from build123d import *

# Parameters (mm, degrees)
BOSS_EXTRUDE1_DEPTH = 5
SKETCH2_W           = 3.3
SKETCH2_H           = 6
CUT_EXTRUDE2_DEPTH  = 6.5
SKETCH3_R           = 2.15
CUT_EXTRUDE4_DEPTH  = 24
FILLET1_R           = 0.5
FILLET2_R           = 3
SKETCH5_W           = 10.2
SKETCH5_H           = 7
CUT_EXTRUDE5_DEPTH  = 44.231932642
SKETCH8_W           = 20
SKETCH8_H           = 7
CUT_EXTRUDE6_DEPTH  = 44.231932642
SKETCH9_W           = 20
SKETCH9_H           = 7
BOSS_EXTRUDE2_DEPTH = 10
SKETCH10_R          = 2.55
CUT_EXTRUDE7_DEPTH  = 45.955533586
FILLET3_R           = 5
SKETCH11_W          = 40
SKETCH11_H          = 10
BOSS_EXTRUDE3_DEPTH = 10
SKETCH13_W          = 35.742737896
SKETCH13_H          = 10
BOSS_EXTRUDE5_DEPTH = 5
SKETCH14_R          = 1.4
CUT_EXTRUDE8_DEPTH  = 47.75467891
SKETCH16_W          = 20
SKETCH16_H          = 3
CUT_EXTRUDE10_DEPTH = 5
SKETCH17_R          = 1
CUT_EXTRUDE11_DEPTH = 3.5


with BuildPart() as part:
    # Sketch1 → Boss-Extrude1 (new, symmetric)
    with BuildSketch(Plane.XY):
        with BuildLine():
            Line((40, -13), (34.35, -13))
            Line((34.35, -13), (34.35, 3))
            ThreePointArc((34.35, 3), (26.182605601, 5.085665361), (32.35, -0.660601044))
            Line((32.35, -0.660601044), (32.35, -13))
            Line((32.35, -13), (7.5, -13))
            Line((7.5, -13), (7.5, -6))
            Line((7.5, -6), (5.1, -6))
            Line((5.1, -6), (5.1, -13))
            Line((5.1, -13), (-5.1, -13))
            Line((-5.1, -13), (-5.1, -6))
            Line((-5.1, -6), (-7.5, -6))
            Line((-7.5, -6), (-7.5, -13))
            Line((-7.5, -13), (-32.35, -13))
            Line((-32.35, -13), (-32.35, -0.660601044))
            ThreePointArc((-32.35, -0.660601044), (-26.182605601, 5.085665361), (-34.35, 3))
            Line((-34.35, 3), (-34.35, -13))
            Line((-34.35, -13), (-40, -13))
            Line((-40, -13), (-40, 13))
            Line((-40, 13), (40, 13))
            Line((40, 13), (40, -13))
        make_face()
    extrude(amount=BOSS_EXTRUDE1_DEPTH, both=True)

    # Sketch2 → Cut-Extrude2 (cut)
    with BuildSketch(Plane.XY.offset(5)):
        with Locations((-24, -10)):
            Rectangle(SKETCH2_W, SKETCH2_H)
        with Locations((24, -10)):
            Rectangle(SKETCH2_W, SKETCH2_H)
    extrude(amount=-CUT_EXTRUDE2_DEPTH, mode=Mode.SUBTRACT)

    # Sketch3 → Cut-Extrude4 (cut)
    with BuildSketch(Plane.ZY.offset(40)):
        with Locations(Location((2, -10, 0), (0, 0, 90))):
            Circle(SKETCH3_R)
    cut_extrude4 = extrude(amount=-CUT_EXTRUDE4_DEPTH, mode=Mode.SUBTRACT)

    # Mirror1: Cut-Extrude4 across plane
    add(cut_extrude4.mirror(Plane(origin=(0, 0, 0), x_dir=(0, 0, 1), z_dir=(1, 0, 0))), mode=Mode.SUBTRACT)

    # Fillet1
    fillet1_edges = [part.edges().sort_by_distance(p)[0] for p in [
        (5.1, -9.5, -5),
        (-5.1, -9.5, -5),
    ]]
    fillet(fillet1_edges, radius=FILLET1_R)

    # Fillet2
    fillet2_edges = [part.edges().sort_by_distance(p)[0] for p in [
        (-40, 13, 0),
        (40, 13, 0),
    ]]
    fillet(fillet2_edges, radius=FILLET2_R)

    # Sketch5 → Cut-Extrude5 (cut, through all)
    with BuildSketch(Plane.XY.offset(5)):
        with Locations((0, -9.5)):
            Rectangle(SKETCH5_W, SKETCH5_H)
    extrude(amount=-CUT_EXTRUDE5_DEPTH, mode=Mode.SUBTRACT)

    # Sketch8 → Cut-Extrude6 (cut, through all)
    with BuildSketch(Plane(origin=(0, 0, -5), x_dir=(-1, 0, 0), z_dir=(0, 0, -1))):
        with Locations((0, -9.5)):
            Rectangle(SKETCH8_W, SKETCH8_H)
    extrude(amount=-CUT_EXTRUDE6_DEPTH, mode=Mode.SUBTRACT)

    # Sketch9 → Boss-Extrude2 (add)
    with BuildSketch(Plane.XY.offset(5)):
        with Locations((0, -2.5)):
            Rectangle(SKETCH9_W, SKETCH9_H)
    extrude(amount=BOSS_EXTRUDE2_DEPTH)

    # Sketch10 → Cut-Extrude7 (cut, through all)
    with BuildSketch(Plane(origin=(0, 1, 0), x_dir=(1, 0, 0), z_dir=(0, 1, 0))):
        with Locations(Location((0, -9.5, 0), (0, 0, 270))):
            Circle(SKETCH10_R)
    extrude(amount=-CUT_EXTRUDE7_DEPTH, mode=Mode.SUBTRACT)

    # Fillet3
    fillet3_edges = [part.edges().sort_by_distance(p)[0] for p in [
        (-10, -2.5, 15),
        (10, -2.5, 15),
    ]]
    fillet(fillet3_edges, radius=FILLET3_R)

    # Sketch11 → Boss-Extrude3 (add)
    with BuildSketch(Plane(origin=(0, 0, -5), x_dir=(-1, 0, 0), z_dir=(0, 0, -1))):
        with Locations((0, -1)):
            Rectangle(SKETCH11_W, SKETCH11_H)
    extrude(amount=BOSS_EXTRUDE3_DEPTH)

    # Sketch13 → Boss-Extrude5 (add)
    with BuildSketch(Plane.XZ.offset(13)):
        Rectangle(SKETCH13_W, SKETCH13_H)
    extrude(amount=BOSS_EXTRUDE5_DEPTH)

    # Sketch14 → Cut-Extrude8 (cut, through all)
    with BuildSketch(Plane.XZ.offset(6)):
        with Locations((-15, -10)):
            Circle(SKETCH14_R)
        with Locations(Location((15, -10, 0), (0, 0, 270))):
            Circle(SKETCH14_R)
    extrude(amount=-CUT_EXTRUDE8_DEPTH, mode=Mode.SUBTRACT)

    # Sketch16 → Cut-Extrude10 (cut)
    with BuildSketch(Plane.XY.offset(5)):
        with Locations((0, -14.5)):
            Rectangle(SKETCH16_W, SKETCH16_H)
    extrude(amount=-CUT_EXTRUDE10_DEPTH, mode=Mode.SUBTRACT)

    # Sketch17 → Cut-Extrude11 (cut)
    with BuildSketch(Plane.XZ.offset(18)):
        with Locations((-13.871368948, 0)):
            Circle(SKETCH17_R)
        with Locations(Location((13.871368948, 0, 0), (0, 0, 180))):
            Circle(SKETCH17_R)
    extrude(amount=-CUT_EXTRUDE11_DEPTH, mode=Mode.SUBTRACT)


solid = part.part
Design review of the part built by this model. Coordinates are the model's own, in mm. A direction names the side the tool comes from. Round coordinates to 2 decimals unless told otherwise and drop trailing zeros. Loops run counter-clockwise (first coordinate to the right, second up) from the corner with the lowest first, then second, coordinate; pieces in that order, holes last. Notation, with made-up numbers: (-29, 28.25) - (-4, 28.25) arc R29 cw to (-4, 62.25) - close; hole circle Ø4 at (-39, 0). An arc over 180 degrees is marked (long way). One line per item, written item: value. Start each with the question number.
1) Draft analysis for pull direction X (two halves, no side actions). For faces 1 (the cylindrical face through (-15.303, -1.07, -11.367)), 2 (the cylindrical face through (39.14, 12.1, 0.07)), 3 (the flat face through (-40, -2, 0)), state which applies: +X half, -X half, draft (parallel to the pull), parting line (faces both ways), or undercut.
2) To check wall thickness, follow L1, parallel to Z at x = 30, y = -10; L2, parallel to X at y = -3.5, z = 1.75; L3, parallel to Y at x = -8, z = -1.75. State the ranges of each line that lie inside material, in increasing order. Write a range as from..to.
3) Consider section A-A on x = 30. Give the boundary of the cut face in (y, z), then the cut area to 3 significant figures.
4) Insertion check: pin 1 Ø1 at (x, z) = (1.5, 11.5) entering from +Y; pin 2 Ø3.5 at (x, y) = (23.5, -10.5) entering from +Z; pin 3 Ø6 at (x, z) = (36, 2) entering from -Y. Each pin has a flat end and moves straight along its axis. Give the tip position at first contact, or say it passes through.
5) Consider section D-D on z = 3. Give the number of separate pieces and of enclosed holes in the cut face, then the cut area to 3 significant figures.
6) Consider section B-B on x = 0. Give the boundary of the cut face in (y, z), then the cut area to 3 significant figures.
7) For faces 4 (the cylindrical face through (19.22, -7.95, 1.35)), 5 (the flat face through (-0.1, 1, 12.2)), 6 (the flat face through (-24, -7, 2)), list the 3-axis set-ups (+Z, -Z, +X, -X, +Y, -Y) from which the entire face can be reached by the end or side of a thin tool; tool diameter is ignored.
8) Consider section C-C on x = 11. Give the boundary of the cut face in (y, z).
Reported:
1. face 1: undercut
1. face 2: +X half
1. face 3: -X half
2. L1: z = -5..-0.15, 4.15..5
2. L2: x = -40..-34.35, -32.35..32.35, 34.35..40
2. L3: y = -18..-13, -6..13
3. outline: (-13, -5) - (-1.35, -5) - (-1.35, 5) - (-13, 5) - close; (7.35, -5) - (13, -5) - (13, 5) - (7.35, 5) - close; hole circle Ø4.3 at (-10, 2)
3. area: 158 mm^2
4. pin 1: stops at y = 1
4. pin 2: stops at z = 5
4. pin 3: stops at y = -13
5. separate pieces: 5
5. enclosed holes: 1
5. area: 1,700 mm^2
6. outline: (-18, -5) - (-13, -5) - (-13, 0) - (-16, 0) - (-16, 5) - (-18, 5) - close; (-6, -15) - (4, -15) - (4, -5) - (13, -5) - (13, 5) - (1, 5) - (1, 6.95) - (-6, 6.95) - close; (-6, 12.05) - (1, 12.05) - (1, 15) - (-6, 15) - close
6. area: 359 mm^2
7. face 4: +X
7. face 5: +Z, +X, -X, +Y
7. face 6: +Z, -Y
8. outline: (-18, -5) - (-6, -5) - (-6, -15) - (4, -15) - (4, -5) - (13, -5) - (13, 5) - (-18, 5) - close
